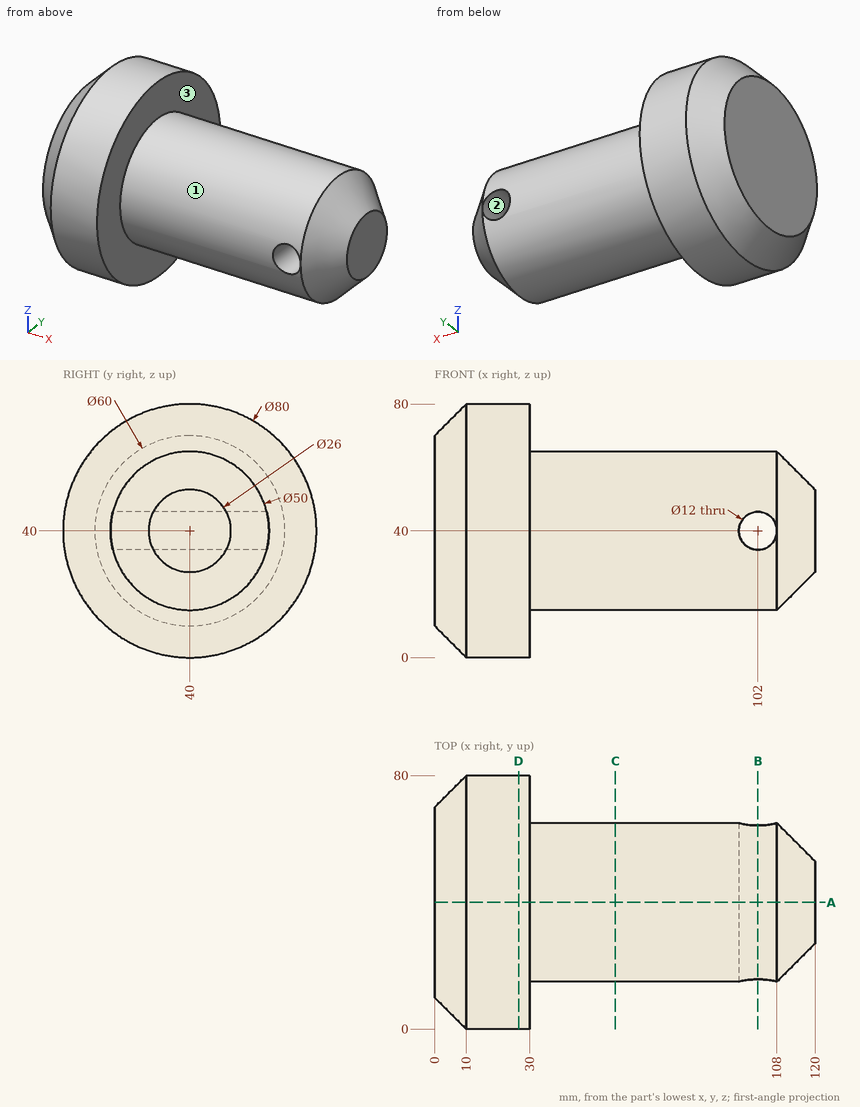
Source: three-view drawing plus pictorial views. Frame: mm from the lowest corner of the part. Give positions to 0.01 mm unless a question says otherwise; leave off trailing zeros. Write each loop counter-clockwise with the first axis right and the second up, starting at its lowest first coordinate (ties: lowest second). Pieces come first, ordered by that corner, then holes. Notation, with made-up numbers: (10, -25) - (42, -25) arc R18 ccw to (42, -19) - close; hole circle Ø10 at (67.25, 32.25). An arc over 180 degrees is marked (long way). Write item = value, one per line. Start each with the question number.
Q1. Cut plane B-B, the plane x = 102. Return loops of the section in (y, z).
Q2. Pin query (flat end, axial travel): pin 1 Ø2 at (y, z) = (28.5, 69) entering from -X; pin 2 Ø2 at (x, z) = (25.5, 22.5) entering from -Y; pin 3 Ø5 at (y, z) = (26, 69) entering from +X. Return the tip coordinate at first contact, or that it passes through.
Q3. Cut plane C-C, the plane x = 57. Return loops of the section in (y, z).
Q4. Cut plane A-A, the plane y = 40. Return loops of the section in (x, z), then the cut area to 3 significant figures.
Q5. Material intervals for probe 1 along X at (y, z) = (33, 40); probe 2 along Z at (x, y) = (102, 29); probe 3 along Z at (x, y) = (102, 47), sorted ascending.
Q6. Cut plane D-D, the plane x = 26.5. Return loops of the section in (y, z), then the cut area to 3 significant figures.
Q7. Draft query along Z for the marked faces 1, 2 and 3. Return one class per face: +Z half, -Z half, draft (parallel to the pull), parting line (faces both ways), or undercut.
Computed values:
q1.outline = (15.73, 34) arc R25 ccw to (64.27, 34) - close; (15.73, 46) - (64.27, 46) arc R25 ccw to start
q2.pin_1 = 0.2
q2.pin_2 = 3.56
q2.pin_3 = 30
q3.outline = circle Ø50 at (40, 40)
q4.outline = (0, 10) - (10, 0) - (30, 0) - (30, 15) - (108, 15) - (120, 27) - (120, 53) - (108, 65) - (30, 65) - (30, 80) - (10, 80) - (0, 70) - close; hole circle Ø12 at (102, 40)
q4.area = 6,540 mm²
q5.probe_1 = 0 to 96, 108 to 120
q5.probe_2 = 17.55 to 34, 46 to 62.45
q5.probe_3 = 16 to 34, 46 to 64
q6.outline = circle Ø80 at (40, 40)
q6.area = 5,030 mm²
q7.face_1 = parting line
q7.face_2 = undercut
q7.face_3 = draft
